Here's how the part is built. I have some questions about the finished solid (model axes, mm). Give positions to 0.01 mm unless a question says otherwise; leave off trailing zeros. Loops run counter-clockwise (first coordinate to the right, second up) from the corner with the lowest first, then second, coordinate; pieces in that order, holes last. Notation, with made-up numbers: (54.25, 22.25) - (79.25, 22.25) arc R20 cw to (79.25, 29.25) - close; hole circle Ø6 at (-28.5, 45). An arc over 180 degrees is marked (long way). Return JSON: item names as keys, results as strings. Group by question number.
(1) If we section it at A-A (x = -25): Please give me the cut outline in (y, z).
(2) For P1, Ø6.5, axis at x = 75, y = 0, coming from the -Z side, with a flat end and sliding along its axis, tell me the tip position at first contact or that it passes through.
(3) If we section it at D-D (x = 17): Please give me the cut outline in (y, z).
(4) If we section it at B-B (z = 1.7): State how many separate pieces and enclosed holes the cut face has, then the cut area to 3 significant figures.
(5) If we section it at C-C (y = 2.25): Please give me the cut outline in (x, z).
(6) I need wall thicknesses on probe 1 along Y at (x, z) = (35.5, 3.15); probe 2 along Y at (x, z) = (75, 1.8); probe 3 along X at (y, z) = (0.5, 0.6). Which ranges of each line are inside material? Lowest first, please. Write a range as [from, to].
```python
from build123d import *

# Parameters (mm, degrees)
SKETCH1_R           = 5.5
BOSS_EXTRUDE1_DEPTH = 5
SKETCH2_W           = 30
SKETCH2_H           = 8
CUT_EXTRUDE1_DEPTH  = 10
FILLET1_R           = 4


with BuildPart() as part:
    # Sketch1 → Boss-Extrude1 (new body)
    with BuildSketch(Plane.XY):
        with BuildLine():
            Line((75, 12.5), (-75, 12.5))
            ThreePointArc((-75, 12.5), (-87.5, 0), (-75, -12.5))
            Line((-75, -12.5), (75, -12.5))
            ThreePointArc((75, -12.5), (87.5, 0), (75, 12.5))
        make_face()
        with Locations((-75, 0)):
            Circle(SKETCH1_R, mode=Mode.SUBTRACT)
        with Locations(Location((75, 0, 0), (0, 0, 180))):
            Circle(SKETCH1_R, mode=Mode.SUBTRACT)
    extrude(amount=BOSS_EXTRUDE1_DEPTH)

    # Sketch2 → Cut-Extrude1 (cut)
    with BuildSketch(Plane(origin=(0, 0, 0), x_dir=(-1, 0, 0), z_dir=(0, 0, -1))):
        with Locations((-30, 0)):
            Rectangle(SKETCH2_W, SKETCH2_H)
        with Locations((30, 0)):
            Rectangle(SKETCH2_W, SKETCH2_H)
    extrude(amount=-CUT_EXTRUDE1_DEPTH, mode=Mode.SUBTRACT)

    # Fillet1
    fillet1_edges = [part.edges().sort_by_distance(p)[0] for p in [
        (15, -4, 2.5),
        (45, -4, 2.5),
        (45, 4, 2.5),
        (15, 4, 2.5),
        (-45, -4, 2.5),
        (-15, -4, 2.5),
        (-15, 4, 2.5),
        (-45, 4, 2.5),
    ]]
    fillet(fillet1_edges, radius=FILLET1_R - 0.0001)  # a hair under: the kernel refuses the full size


solid = part.part
```
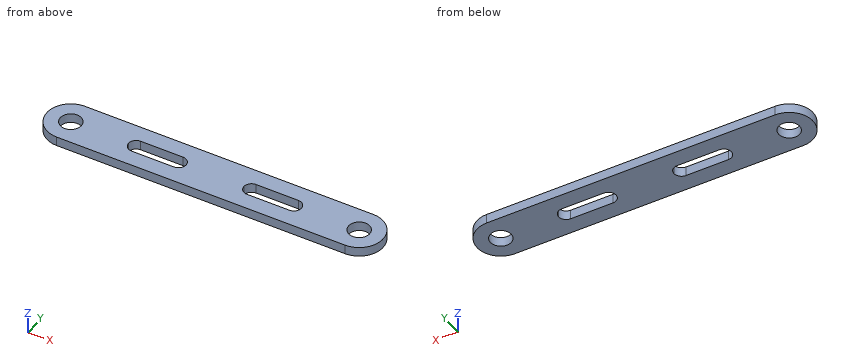
Values:
{
 "1": {"outline": "(-12.5, 0) - (-4, 0) - (-4, 5) - (-12.5, 5) - close; (4, 0) - (12.5, 0) - (12.5, 5) - (4, 5) - close"},
 "2": {"P1": "through"},
 "3": {"outline": "(-12.5, 0) - (-3.46, 0) - (-3.46, 5) - (-12.5, 5) - close; (3.46, 0) - (12.5, 0) - (12.5, 5) - (3.46, 5) - close"},
 "4": {"separate pieces": "1", "enclosed holes": "4", "area": "3,600 mm2"},
 "5": {"outline": "(-87.3, 0) - (-80.02, 0) - (-80.02, 5) - (-87.3, 5) - close; (-69.98, 0) - (-44.31, 0) - (-44.31, 5) - (-69.98, 5) - close; (-15.69, 0) - (15.69, 0) - (15.69, 5) - (-15.69, 5) - close; (44.31, 0) - (69.98, 0) - (69.98, 5) - (44.31, 5) - close; (80.02, 0) - (87.3, 0) - (87.3, 5) - (80.02, 5) - close"},
 "6": {"probe 1": "[-12.5, -4], [4, 12.5]", "probe 2": "[-12.5, -5.5], [5.5, 12.5]", "probe 3": "[-87.49, -80.48], [-69.52, -44.97], [-15.03, 15.03], [44.97, 69.52], [80.48, 87.49]"}
}
